```python
from build123d import *

# Parameters (mm, degrees)
SKETCH9_W           = 300
SKETCH9_H           = 590
SKETCH9_W_2         = 187.325
SKETCH9_H_2         = 265.1125
BOSS_EXTRUDE7_DEPTH = 3.175
FILLET4_R           = 10
FILLET5_R           = 12.7


with BuildPart() as part:
    # Sketch9 → Boss-Extrude7 (new body)
    with BuildSketch(Plane(origin=(0, 0, 0), x_dir=(1, 0, 0), z_dir=(0, 1, 0))):
        with Locations((0, 275)):
            Rectangle(SKETCH9_W, SKETCH9_H)
        with Locations((-10, 290)):
            Rectangle(SKETCH9_W_2, SKETCH9_H_2, mode=Mode.SUBTRACT)
    extrude(amount=BOSS_EXTRUDE7_DEPTH)

    # Fillet4
    fillet4_edges = [part.edges().sort_by_distance(p)[0] for p in [
        (150, 1.5875, -570),
        (150, 1.5875, 20),
        (-150, 1.5875, 20),
        (-150, 1.5875, -570),
    ]]
    fillet(fillet4_edges, radius=FILLET4_R)

    # Fillet5
    fillet5_edges = [part.edges().sort_by_distance(p)[0] for p in [
        (83.6625, 1.5875, -157.44375),
        (83.6625, 1.5875, -422.55625),
        (-103.6625, 1.5875, -422.55625),
        (-103.6625, 1.5875, -157.44375),
    ]]
    fillet(fillet5_edges, radius=FILLET5_R)


solid = part.part
```
The listing builds one solid part. Answer for the finished solid, in the listing's coordinates (mm). A direction names the side the tool comes from. Coordinates: 2 decimals unless noted, no trailing zeros. Loops run counter-clockwise (first coordinate to the right, second up) from the corner with the lowest first, then second, coordinate; pieces in that order, holes last. Notation, with made-up numbers: (-1, -16) - (39, -16) arc R11 ccw to (39, -3) - close; hole circle Ø10 at (45, 22.5). An arc over 180 degrees is marked (long way). Use a Markdown table: item, result. Add a question column.
1) The part is cut by section B-B, the plane z = -231.5. Give the vertices of the cut face in (x, y) (1 decimal).
2) The part is cut by section A-A, the plane x = -72. Give the vertices of the cut face in (y, z) (3 decimals).
3) For faces 1 (the cylindrical face through (-99.843, 1.61, -161.065)), 2 (the cylindrical face through (146.99, 1.61, -567.15)), determine the directions among +Z, -Z, +X, -X, +Y, -Y from which every point of the face is accessible in a straight line to the end or side of a thin tool.
4) Find the intervals of material crossed by line 1 (Z direction, x = -15, y = 1.2); line 2 (X direction, y = 1.95, z = -339); line 3 (Z direction, x = 77.5, y = 1), in increasing order.
5) The part is cut by section C-C, the plane y = 1.1. Give the vertices of the cut face in (x, z), and give its area (3 significant figures).
6) The mould has two halves that part along Z. Classify faces 3 (the cylindrical face through (-147.15, 1.61, 16.99)), 4 (the flat face through (98, 0, -279)), 5 (the cylindrical face through (-99.843, 1.61, -418.935)): released by +Z, released by -Z, zero draft, split by the parting line, or undercut.
Here are the results:
| question | item | result |
|---|---|---|
| 1 | outline | (-150, 0) - (-103.7, 0) - (-103.7, 3.2) - (-150, 3.2) - close; (83.7, 0) - (150, 0) - (150, 3.2) - (83.7, 3.2) - close |
| 2 | outline | (0, -570) - (3.175, -570) - (3.175, -422.556) - (0, -422.556) - close; (0, -157.444) - (3.175, -157.444) - (3.175, 20) - (0, 20) - close |
| 3 | face 1 | +Y, -Y |
| 3 | face 2 | -Z, +X, +Y, -Y |
| 4 | line 1 | z = -570 to -422.56, -157.44 to 20 |
| 4 | line 2 | x = -150 to -103.66, 83.66 to 150 |
| 4 | line 3 | z = -570 to -420.74, -159.26 to 20 |
| 5 | outline | (-150, -560) arc R10 ccw to (-140, -570) - (140, -570) arc R10 ccw to (150, -560) - (150, 10) arc R10 ccw to (140, 20) - (-140, 20) arc R10 ccw to (-150, 10) - close; hole (-103.66, -409.86) arc R12.7 ccw to (-90.96, -422.56) - (70.96, -422.56) arc R12.7 ccw to (83.66, -409.86) - (83.66, -170.14) arc R12.7 ccw to (70.96, -157.44) - (-90.96, -157.44) arc R12.7 ccw to (-103.66, -170.14) - close |
| 5 | area | 127,000 mm^2 |
| 6 | face 3 | released by +Z |
| 6 | face 4 | zero draft |
| 6 | face 5 | undercut |
